For this review, take the finished solid that the model builds, in its own axes (mm). Face numbers are marked on the shaded views. A direction names the side the tool comes from. Round coordinates to 2 decimals unless told otherwise and drop trailing zeros. Write each loop counter-clockwise with the first axis right and the second up, starting at its lowest first coordinate (ties: lowest second). Pieces come first, ordered by that corner, then holes. Notation, with made-up numbers: M -11,81.25 L 33,81.25 A23 ccw 33,112.25 Z; hole C -6,13.25 d4. An arc over 180 degrees is marked long. Answer in a Markdown table with one row per item.
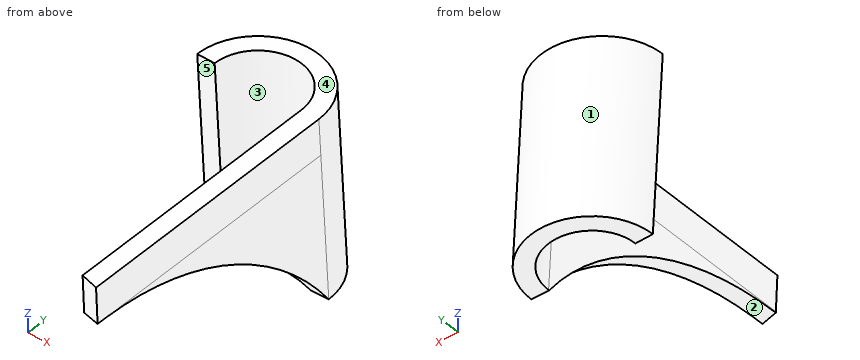
```python
from build123d import *

# Parameters (mm, degrees)
SKETCH1_R               = 3.2639
BOSS_EXTRUDE1_DEPTH     = 10
SKETCH2_W               = 55.96454122
SKETCH2_H               = 39.556429901
BOSS_EXTRUDE2_DEPTH     = 50
CUT_EXTRUDE1_DEPTH      = 3.621876658
CUT_EXTRUDE1_DEPTH_BACK = 57.750909587
CUT_EXTRUDE3_DEPTH      = 104.020815944
BOSS_EXTRUDE3_REACH     = 105.021
SKETCH10_R              = 90
CUT_EXTRUDE4_DEPTH      = 50
CUT_EXTRUDE5_DEPTH      = 50


with BuildPart() as part:
    # Sketch1 → Boss-Extrude1 (new body)
    with BuildSketch(Plane.XY):
        with BuildLine():
            ThreePointArc((0, -23.8125), (-4.393398282, -34.419101718), (-15, -38.8125))
            Line((-15, -38.8125), (-119.778475404, -10.737192131))
            Line((-119.778475404, -10.737192131), (-119.778475404, 66.887807869))
            Line((-119.778475404, 66.887807869), (-15, 38.8125))
            ThreePointArc((-15, 38.8125), (-4.393398282, 34.419101718), (0, 23.8125))
            Line((0, 23.8125), (0, -23.8125))
        make_face()
        with Locations((-15, 23.8125)):
            Circle(SKETCH1_R, mode=Mode.SUBTRACT)
        with Locations((-15, -23.8125)):
            Circle(SKETCH1_R, mode=Mode.SUBTRACT)
    extrude(amount=BOSS_EXTRUDE1_DEPTH)

    # Sketch2 → Boss-Extrude2 (add)
    with BuildSketch(Plane.XY.offset(10)):
        with Locations((-137.760746014, 83.986530895)):
            Rectangle(SKETCH2_W, SKETCH2_H)
    extrude(amount=-BOSS_EXTRUDE2_DEPTH)

    # Sketch4 → Cut-Extrude1 (cut, two sides)
    with BuildSketch(Plane(origin=(-0.959208406, 0, 16.788657247), x_dir=(0, 1, 0), z_dir=(-0.057041289, 0, 0.99837182))) as cut_extrude1_sk:
        with BuildLine():
            ThreePointArc((64.208315944, 114.013041626), (81.708315944, 131.513041626), (64.208315944, 149.013041626))
            Line((64.208315944, 149.013041626), (64.208315944, 176.700065815))
            Line((64.208315944, 176.700065815), (111.984574651, 176.700065815))
            Line((111.984574651, 176.700065815), (111.984574651, 106.901315277))
            Line((111.984574651, 106.901315277), (64.208315944, 106.901315277))
            Line((64.208315944, 106.901315277), (64.208315944, 114.013041626))
        make_face()
        with BuildLine():
            Line((64.208315944, 144.013041626), (64.208315944, 119.013041626))
            ThreePointArc((64.208315944, 119.013041626), (76.708315944, 131.513041626), (64.208315944, 144.013041626))
        make_face()
    extrude(amount=CUT_EXTRUDE1_DEPTH, mode=Mode.SUBTRACT)
    extrude(cut_extrude1_sk.sketch, amount=-CUT_EXTRUDE1_DEPTH_BACK, mode=Mode.SUBTRACT)

    # Sketch7 → Cut-Extrude3 (cut, through all)
    with BuildSketch(Plane(origin=(0, 64.208315944, 0), x_dir=(1, 0, 0), z_dir=(0, 1, 0))):
        Polygon((-119.778475404, 0), (-119.207132269, 0), (-119.778475404, -10), align=None)
    extrude(amount=-CUT_EXTRUDE3_DEPTH, mode=Mode.SUBTRACT)

    # Boss-Extrude3: up to this face of the body (flat: up to its plane)
    boss_extrude3_end = Plane(part.part.faces().sort_by_distance((-67.246532084, -24.813083921, 5.004556479))[0])
    # Sketch8 → Boss-Extrude3 (add, up to the picked face)
    with BuildSketch(Plane.XZ.offset(-64.208315944), mode=Mode.PRIVATE) as boss_extrude3_sk1:
        Polygon((-119.207132269, 0), (-116.92175973, -40), (-111.913605554, -40), (-114.198978093, 0), align=None)
    boss_extrude3_tool1 = split(extrude(boss_extrude3_sk1.sketch, amount=BOSS_EXTRUDE3_REACH, mode=Mode.PRIVATE), bisect_by=boss_extrude3_end, keep=Keep.BOTH, mode=Mode.PRIVATE)
    add(boss_extrude3_tool1.solids().sort_by_distance((-115.560369, 64.208316, -20))[0])

    # Sketch10 → Cut-Extrude4 (cut)
    with BuildSketch(Plane(origin=(-113.827407897, 0, -6.503450805), x_dir=(0.057041289, 0, -0.99837182), z_dir=(0.99837182, 0, 0.057041289))):
        with Locations((83.472510719, -10.677332841)):
            Circle(SKETCH10_R)
    extrude(amount=-CUT_EXTRUDE4_DEPTH, mode=Mode.SUBTRACT)

    # Sketch13 → Cut-Extrude5 (cut)
    with BuildSketch(Plane(origin=(-0.959208406, 0, 16.788657247), x_dir=(0, 1, 0), z_dir=(-0.057041289, 0, 0.99837182))):
        Polygon((64.208315944, 114.013041626), (-14.406743592, 114.013041626), (-68.138706229, -11.161425168), (108.567056958, -47.624519159), align=None)
    extrude(amount=-CUT_EXTRUDE5_DEPTH, mode=Mode.SUBTRACT)


solid = part.part
```
Q1. Take a section at B-B (y = 36.5). State the section outline as (x, z) points.
Found:
| item | result |
|---|---|
| outline | M -119.78,10 L -118.43,-13.61 L -113.44,-13.32 L -114.77,10 Z |
Q2. Machinability: for the marked faces 4 and 5, which of the approach directions +Z, -Z, +X, -X, +Y, -Y give a long, thin tool a straight path to every point of the face, cutting with its end or side? Answer none if there is none.
Found:
| item | result |
|---|---|
| face 4 | +Z, +X, -X, +Y, -Y |
| face 5 | +Z, -Z, -X, -Y |
Q3. Take a section at A-A (y = 49). State the section outline as (x, z) points, then the cut area to 3 significant figures.
Found:
| item | result |
|---|---|
| outline | M -119.78,10 L -117.9,-22.87 L -112.91,-22.58 L -114.77,10 Z |
| area | 164 mm² |
Q4. Mouldability with a two-part tool opening along X and no side actions: class the marked faces 1, 2 and 3 as +X half, -X half, draft (parallel to the pull), parting line (faces both ways), or undercut.
Found:
| item | result |
|---|---|
| face 1 | parting line |
| face 2 | +X half |
| face 3 | undercut |
Q5. For probe 1 along X at (y, z) = (72.5, -1); probe 2 along X at (y, z) = (66, -37.5); probe 3 along X at (y, z) = (59, -16), list the stretches that pass through material, from the lowest coordinate up.
Found:
| item | result |
|---|---|
| probe 1 | -147.11 to -141.04, -122.3 to -116.23 |
| probe 2 | -147.02 to -141.98, -117.19 to -112.15 |
| probe 3 | -118.29 to -113.28 |
Q6. Insertion check: P1, Ø6.5, axis at x = -145, z = -26, coming from the -Y side; P2, Ø4, axis at y = 46, z = -6, coming from the +X side; P3, Ø10, axis at y = 33, z = -10, coming from the -X side. Each pin has a flat end and moves straight along its axis. Give the tip position at first contact, or say it passes through.
Found:
| item | result |
|---|---|
| P1 | y = 64.21 |
| P2 | x = -113.74 |
| P3 | x = -118.92 |
